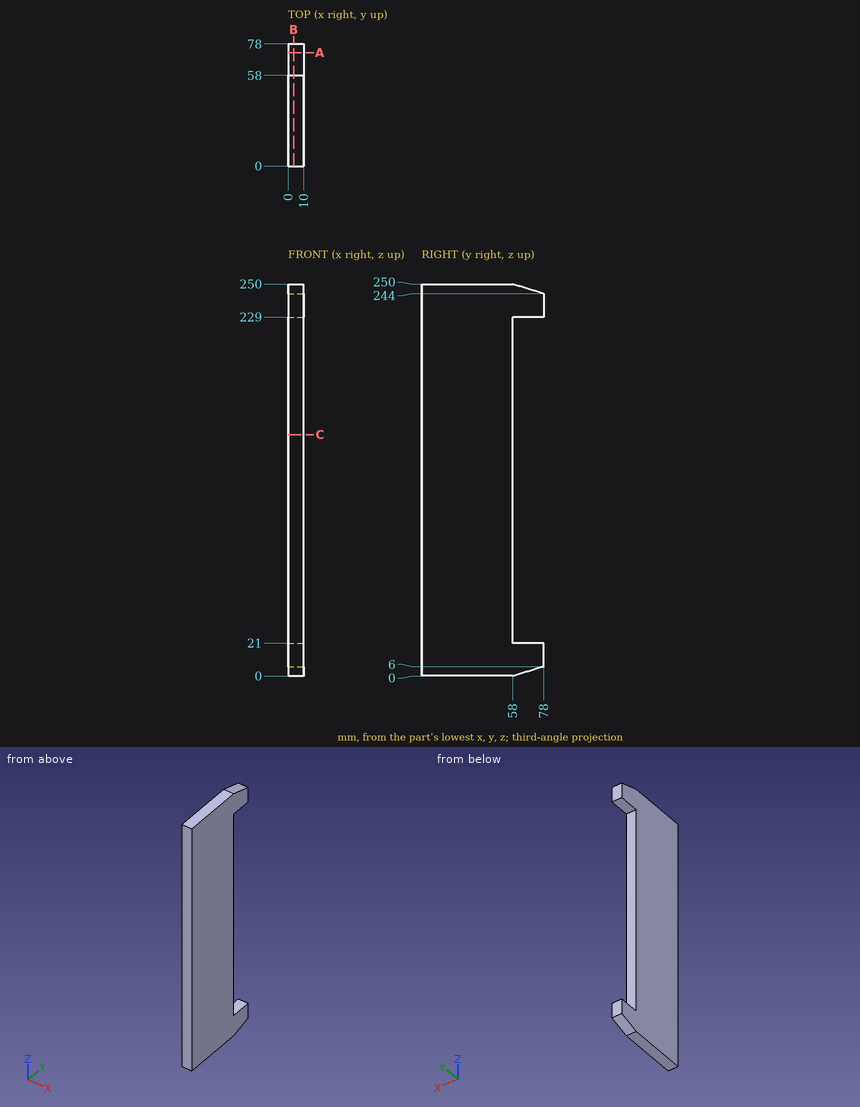
Study the drawing (mm; zero at the part's minimum x, y, z) and answer. Coordinates: 2 decimals unless noted, no trailing zeros. Order: outer loops, then holes, each group sorted by start corner. A loop starts at its lowest first (then second) coordinate and runs counter-clockwise, first axis right, second up. Notation, with made-up numbers: (30.25, 51) -> (38.25, 51) arc R19 cw to (38.25, 61) -> close; hole circle Ø10 at (9.25, 29.5). An arc over 180 degrees is marked (long way). Answer in a Markdown table with one row per item. Add a question column.
Item 1: Find section C-C (z = 154). Write down the section's boundary in (x, y).
Item 2: Find the intervals of material crossed by L1, parallel to Y at x = 7.75, z = 63; L2, parallel to Z at x = 7.75, y = 59, in increasing order. Write a range as from..to.
Item 3: Find section A-A (y = 72.5). Write down the section's boundary in (x, z).
Item 4: Find section B-B (x = 3.5). Write down the section's boundary in (y, z).
Item 5: Each of these flat-tipped pins is pushed along its axis until it touches: P1, Ø5, axis at x = 7, y = 63, coming from the -Z side; P2, Ø2, axis at x = 7.5, z = 128.5, coming from the +Y side; P3, Ø5, axis at x = 3, y = 65, coming from the +Z side. Where does it stop, or does it pass through?
Result set:
| question | item | result |
|---|---|---|
| 1 | outline | (0, 0) -> (10, 0) -> (10, 58) -> (0, 58) -> close |
| 2 | L1 | y = 0..58 |
| 2 | L2 | z = 0.3..21, 229..249.7 |
| 3 | outline | (0, 4.35) -> (10, 4.35) -> (10, 21) -> (0, 21) -> close; (0, 229) -> (10, 229) -> (10, 245.65) -> (0, 245.65) -> close |
| 4 | outline | (0, 0) -> (58, 0) -> (78, 6) -> (78, 21) -> (58, 21) -> (58, 229) -> (78, 229) -> (78, 244) -> (58, 250) -> (0, 250) -> close |
| 5 | P1 | stops at z = 0.75 |
| 5 | P2 | stops at y = 58 |
| 5 | P3 | stops at z = 248.65 |
